Build history of the part. All positions in model axes, mm. Face numbers are marked on the shaded views. Coordinates: 2 decimals unless noted, no trailing zeros. Order: outer loops, then holes, each group sorted by start corner. A loop starts at its lowest first (then second) coordinate and runs counter-clockwise, first axis right, second up. Notation, with made-up numbers: (39, 38.25) -> (53, 38.25) arc R13 cw to (53, 51.25) -> close; hole circle Ø11 at (26.5, 68). An arc over 180 degrees is marked (long way). Write each question's results on one line, items separated by ' | '.
from build123d import *

# Parameters (mm, degrees)
F4_D           = 4.5
F4_DEPTH       = 25
F4_TIP         = 1.3519363928
F4_ON_F3_D     = 4.5
F4_ON_F3_DEPTH = 25
F4_ON_F3_TIP   = 1.3519363928


with BuildPart() as f1:
    # F0 (on Front) → F1 (revolve)
    with BuildSketch(Plane.XZ):
        Polygon((-65, 7.5), (-65, 0), (65, 0), (65, 7.5), (59.4019237886, 6), (-59.4019237886, 6), align=None)
    revolve(axis=Axis((0, 0, 0), (-1, 0, 0)))

    # F4
    with Locations(Plane(origin=(-65, 0, 0), x_dir=(0, -1, 0), z_dir=(-1, 0, 0))):
        with Locations((0, 0)):
            Hole(F4_D / 2, depth=F4_DEPTH)
            with Locations((0, 0, -(F4_DEPTH + F4_TIP / 2))):  # 118° drill point
                Cone(0, F4_D / 2, F4_TIP, mode=Mode.SUBTRACT)

    # F4 on F3
    with Locations(Plane.YZ.offset(65)):
        with Locations((0, 0)):
            Hole(F4_ON_F3_D / 2, depth=F4_ON_F3_DEPTH)
            with Locations((0, 0, -(F4_ON_F3_DEPTH + F4_ON_F3_TIP / 2))):  # 118° drill point
                Cone(0, F4_ON_F3_D / 2, F4_ON_F3_TIP, mode=Mode.SUBTRACT)


solid = f1.part
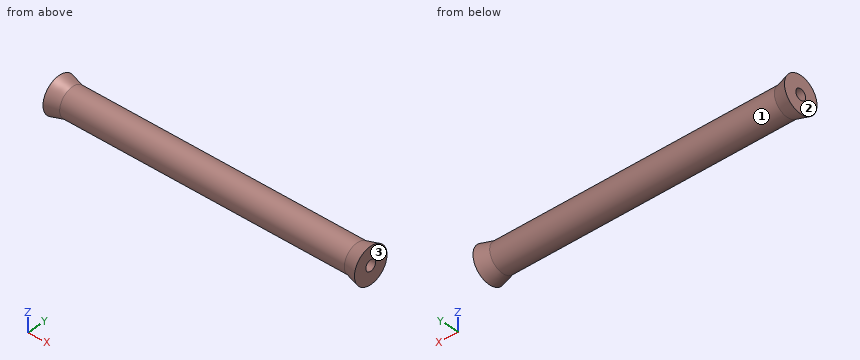
Item 1: Drill centre lines: line 1 (Y direction, x = 55, z = 0); line 2 (Y direction, x = -47, z = -0.75); line 3 (Z direction, x = 51, y = -0.25). Where is each one in solid material? Low to high. Write a range as from..to.
Answer:
line 1: y = -6..-2.25, 2.25..6 | line 2: y = -5.95..-2.12, 2.12..5.95 | line 3: z = -5.99..-2.24, 2.24..5.99
Item 2: Pin check, flat tips, straight feed: pin 1 (1 mm diameter, centred on x = -19.5, z = 0.5, fed in from +Y); pin 2 (4 mm diameter, centred on x = 44, y = -2, fed in from +Z); pin 3 (2.5 mm diameter, centred on y = 0, z = 0, fed in from -X). Stop position of each tip, or through.
Answer:
pin 1: stops at y = 6 | pin 2: stops at z = 6 | pin 3: stops at x = -39.4
Item 3: Pull direction X, two halves, no side cores. Call the marked faces 1, 2 and 3: released by +X, released by -X, zero draft, split by the parting line, or undercut.
Answer:
face 1: undercut | face 2: released by -X | face 3: released by +X
Item 4: Slice it at A-A, the plane x = -8. List the corners of the cut face in (y, z), and give its area (3 significant figures).
Answer:
outline: circle Ø12 at (0, 0) | area: 113 mm^2
